The model under review builds one solid part; all positions refer to its coordinate system, in mm. A direction names the side the tool comes from. Give positions to 0.01 mm unless a question says otherwise; leave off trailing zeros. Loops run counter-clockwise (first coordinate to the right, second up) from the corner with the lowest first, then second, coordinate; pieces in that order, holes last. Notation, with made-up numbers: M 65,76.5 L 97,76.5 A20 cw 97,112.5 Z; hole C 60.25,-22 d10. An arc over 180 degrees is marked long. Put each result on its own line as item: value. Start each with the question number.
```python
from build123d import *

# Parameters (mm, degrees)
F0_W      = 23
F0_H      = 10
F1_DEPTH  = 8
F2_R      = 4.000122
F3_DEPTH  = 5
F4_R      = 12.513681
F5_DEPTH  = 1.5
F6_R      = 3.667742
F7_DEPTH  = 8
F8_R      = 3.62132
F10_DEPTH = 25
F13_DEPTH = 25
F14_W     = 28.555372
F14_H     = 6.345639
F15_DEPTH = 9.5


with BuildPart() as f1:
    # F0 (on Right) → F1 (new body)
    with BuildSketch(Plane.YZ):
        Rectangle(F0_W, F0_H)
    extrude(amount=F1_DEPTH)

    # F2 (on face) → F3 (join)
    with BuildSketch(Plane.XZ.offset(11.5)):
        with Locations((3.999878, 0)):
            Circle(F2_R)
    extrude(amount=F3_DEPTH)

    # F4 (on face) → F5 (join)
    with BuildSketch(Plane.XZ.offset(16.5)):
        with Locations((3.999878, 0)):
            Circle(F4_R)
    extrude(amount=F5_DEPTH)

    # F6 (on face) → F7 (join)
    with BuildSketch(Plane.XZ.offset(18)):
        with Locations((3.999878, 0)):
            Circle(F6_R)
    extrude(amount=F7_DEPTH)

    # F8
    f8_edges = [f1.edges().sort_by_distance(p)[0] for p in [
        (0.332136, -26, 0),
    ]]
    fillet(f8_edges, radius=F8_R)

    # F9 (on face) → F10 (cut)
    with BuildSketch(Plane.XY.offset(5)):
        with BuildLine():
            ThreePointArc((4, -1.300277), (4.919435, -0.919435), (5.300277, 0))
            ThreePointArc((5.300277, 0), (3.080565, 0.919435), (4, -1.300277))
        make_face()
    extrude(amount=-F10_DEPTH, mode=Mode.SUBTRACT)

    # F11 (on face) → F13 (cut)
    with BuildSketch(Plane.XY.offset(5)):
        with BuildLine():
            ThreePointArc((4, -5.995241), (4.919239, -5.61448), (5.3, -4.695241))
            ThreePointArc((5.3, -4.695241), (3.080761, -3.776003), (4, -5.995241))
        make_face()
    extrude(amount=-F13_DEPTH, mode=Mode.SUBTRACT)

    # F14 (on face) → F15 (cut)
    with BuildSketch(Plane(origin=(0, 0, -5), x_dir=(1, 0, 0), z_dir=(0, 0, -1))):
        with Locations((3.811784, 17.208513)):
            Rectangle(F14_W, F14_H)
    extrude(amount=F15_DEPTH, mode=Mode.SUBTRACT)


solid = f1.part
```
Item 1: To check wall thickness, follow L1, parallel to Y at x = 4, z = 1; L2, parallel to X at y = 0, z = 0; L3, parallel to Y at x = 4, z = 1.75. State the ranges of each line that lie inside material, in increasing order. Write a range as [from, to].
Item 2: Draft analysis for pull direction Y (two halves, no side actions). For faces 4 (the flat face through (4, -18, 4)), 5 (the flat face through (4, 11.5, 0)), 6 (the flat face through (4, -11.5, 4.2)), state which applies: +Y half, -Y half, draft (parallel to the pull), parting line (faces both ways), or undercut.
Item 3: Consider section A-A, the plane y = 4. Write out the cut boundary in (x, z).
Item 4: Clearance check with flat-ended pins moving along their axes: pin 1 Ø2 at (x, y) = (0.5, -18.5) entering from -Z; pin 2 Ø8 at (y, z) = (1.5, 0.5) entering from -X; pin 3 Ø6.5 at (x, y) = (5.5, 0.5) entering from +Z; pin 4 Ø2.5 at (x, z) = (5, -3.5) entering from -Y. State where each tip first meets the part, or that it passes through.
Item 5: Consider section C-C, the plane x = -5.25. Write out the cut boundary in (y, z), plus the area to 3 significant figures.
Item 6: Tool access review of faces 1 (the cylindrical face through (7.815, -13.965, 1.202)), 2 (the flat face through (8, 0, 0)), 3 (the flat face through (2, 0, 5)): name each direction out of +Z, -Z, +X, -X, +Y, -Y from which nothing blocks a thin tool from reaching the whole face with its end or side.
Item 7: Consider section B-B, the plane z = -3.25. Give the number of separate pieces and of enclosed holes in the cut face, plus the area to 3 significant figures.
Report:
1. L1: [-25.87, -6], [-3.4, -1.3], [1.3, 11.5]
1. L2: [0, 2.7], [5.3, 8]
1. L3: [-25.57, -6], [-3.4, -1.3], [1.3, 11.5]
2. face 4: -Y half
2. face 5: +Y half
2. face 6: undercut
3. outline: M 0,-5 L 8,-5 L 8,5 L 0,5 Z
4. pin 1: z = -5
4. pin 2: x = 0
4. pin 3: z = 5
4. pin 4: y = -25.14
5. outline: M -18,-5 L -16.5,-5 L -16.5,8.43 L -18,8.43 Z
5. area: 20.1 mm²
6. face 1: none
6. face 2: +Z, -Z, +X, +Y
6. face 3: +Z, +X, -X, +Y
7. separate pieces: 1
7. enclosed holes: 2
7. area: 252 mm²
